Source: CAD feature listing. Evaluate the final solid. Frame: model axes, mm. A direction names the side the tool comes from. Round coordinates to 2 decimals unless told otherwise and drop trailing zeros. Loops run counter-clockwise (first coordinate to the right, second up) from the corner with the lowest first, then second, coordinate; pieces in that order, holes last.
Item 1: Section query C-C on x = 87. Return loops of the section in (y, z), then the cut area to 3 significant figures.
Item 2: Access query for faces 1 (the flat face through (43.95, 14.44, 15.43)), 2 (the flat face through (43.828, -12.443, 15.57)). Directions: +Z, -Z, +X, -X, +Y, -Y. A direction counts if a zero-diameter tool reaches every point of the face in a straight line with its end or side. Return the directions, or none.
Item 3: First-contact query: P1, Ø6, axis at x = 11, z = 18, coming from the -Y side; P2, Ø1, axis at x = 80.5, z = 13, coming from the +Y side; P3, Ø2, axis at y = 8, z = 18.5, coming from the +X side. Flat tips, straight axial feed; report the tip coordinate or a pass-through.
Item 4: Ray query, L1, parallel to Y at x = 3, z = 15.75; L2, parallel to X at y = -6, z = 13; L3, parallel to X at y = -3, z = 11.75. Return the intervals inside material, ascending.
Item 5: Section query A-A on z = 12.5. Return loops of the section in (x, y).
Item 6: Pull-direction query (Y, two-part tool) for faces 3 (the flat face through (43.828, 12.443, 15.57)), 4 (the flat face through (43.95, -14.44, 15.43)), 5 (the flat face through (39, -14, 10.5)); classes: released by +Y, released by -Y, zero draft, split by the parting line, or undercut.
Item 7: Section query B-B on y = -14. Return loops of the section in (x, z).
```python
from build123d import *

# Parameters (mm, degrees)
SKIZZE2_W = 2
SKIZZE2_H = 10


with BuildPart() as part:
    # Austragung1: sweep along a path in Skizze3
    with BuildLine(Plane.XY.offset(15.5)) as austragung1_path:
        ThreePointArc((-15, 0), (-10.289915109, 10.914103127), (0.882352941, 14.974025955))
        Line((0.882352941, 14.974025955), (85.588235294, 9.98268397))
        ThreePointArc((85.588235294, 9.98268397), (92.276068751, 6.859943406), (95, 0))
    # Skizze2 → Austragung1 (sweep)
    with BuildSketch(Plane(origin=(0, 0, 0), x_dir=(1, 0, 0), z_dir=(0, 1, 0))):
        with Locations((-16, -15.5)):
            Rectangle(SKIZZE2_W, SKIZZE2_H)
    sweep(path=austragung1_path.line)

    # Spiegeln1: part across plane


with BuildPart() as part_1:
    add(part.part)
    add(part.part.mirror(Plane(origin=(0, 0, 0), x_dir=(0, 0, 1), z_dir=(0, -1, 0))))


solid = part_1.part
```
Data:
1. outline: (-11.83, 10.5) - (-9.8, 10.5) - (-9.8, 20.5) - (-11.83, 20.5) - close; (9.8, 10.5) - (11.83, 10.5) - (11.83, 20.5) - (9.8, 20.5) - close
1. area: 40.7 mm2
2. face 1: +Z, -Z, +X, +Y
2. face 2: +Z, -Z
3. P1: stops at y = -16.56
3. P2: stops at y = 12.32
3. P3: stops at x = 94.75
4. L1: y = -16.85 to -14.85, 14.85 to 16.85
4. L2: x = -15.91 to -13.75, 93 to 95.39
4. L3: x = -16.73 to -14.7, 94.54 to 96.62
5. outline: (1, -16.97) - (85.71, -11.98) arc R12 ccw to (85.71, 11.98) - (1, 16.97) arc R17 ccw (long way) to start; hole (0.88, -14.97) - (85.59, -9.98) arc R10 ccw to (85.59, 9.98) - (0.88, 14.97) arc R15 ccw (long way) to start
6. face 3: undercut
6. face 4: released by -Y
6. face 5: zero draft
7. outline: (-9.64, 10.5) - (-5.39, 10.5) - (-5.39, 20.5) - (-9.64, 20.5) - close; (17.41, 10.5) - (51.41, 10.5) - (51.41, 20.5) - (17.41, 20.5) - close
